Here's how the part is built. I have some questions about the finished solid (model axes, mm). A direction names the side the tool comes from. Coordinates: 2 decimals unless noted, no trailing zeros. Loops run counter-clockwise (first coordinate to the right, second up) from the corner with the lowest first, then second, coordinate; pieces in that order, holes last. Notation, with made-up numbers: (-14, 76) -> (33, 76) arc R8 cw to (33, 86) -> close; hole circle Ø11 at (-8, 27.5). An arc over 180 degrees is marked (long way). Use CSV: the item, a comma, the result in double quotes. Start each with the question number.
from build123d import *

# Parameters (mm, degrees)
SKETCH1_W           = 25.4
SKETCH1_H           = 299.72
BOSS_EXTRUDE1_DEPTH = 417.83
SKETCH2_W           = 223.52
SKETCH2_H           = 810.26
CUT_EXTRUDE1_DEPTH  = 19.05
SKETCH3_W           = 25.4
SKETCH3_H           = 118.11
CUT_EXTRUDE2_DEPTH  = 12.7


with BuildPart() as part:
    # Sketch1 → Boss-Extrude1 (new, symmetric)
    with BuildSketch(Plane(origin=(0, 0, 0), x_dir=(1, 0, 0), z_dir=(0, 1, 0))):
        Rectangle(SKETCH1_W, SKETCH1_H)
    extrude(amount=BOSS_EXTRUDE1_DEPTH, both=True)

    # Sketch2 → Cut-Extrude1 (cut)
    with BuildSketch(Plane(origin=(12.7, 0, 0), x_dir=(0, 0, -1), z_dir=(1, 0, 0))):
        Rectangle(SKETCH2_W, SKETCH2_H)
    extrude(amount=-CUT_EXTRUDE1_DEPTH, mode=Mode.SUBTRACT)

    # Sketch3 → Cut-Extrude2 (cut)
    with BuildSketch(Plane.ZY.offset(12.7)):
        with Locations((130.81, 231.775)):
            Rectangle(SKETCH3_W, SKETCH3_H)
    extrude(amount=-CUT_EXTRUDE2_DEPTH, mode=Mode.SUBTRACT)


solid = part.part
1) Which directions (+Z, -Z, +X, -X, +Y, -Y) give clear straight access to the entire face, cutting with the end or side of a thin tool? Please do faces 5 (the face through (3, -405.13, 2)), 6 (the face through (0, 6, -149.86)), 7 (the face through (0, 233, 131)).
2) Thinking about a two-plate mould opening in Y: for faces 1 (the face through (0, 417.83, -2)), 2 (the face through (3, -6, 111.76)), 3 (the face through (3, 405.13, 2)), 4 (the face through (-12.7, 6, 2)), which applies, pulls with the +Y half, pulls with the -Y half, needs draft (parallel to the pull), parting line crosses it, or undercut?
3) Please list where these lines run through material, in increasing order: L1, parallel to Z at x = -1.25, y = 341.5; L2, parallel to Y at x = 11.5, z = 6; L3, parallel to Z at x = -1, y = 262. Write a range as [from, to].
4) I want a section at B-B, the plane y = 279. Please give me the cut outline in (x, z).
5) I want a section at A-A, the plane z = -3.5. Please give me the cut outline in (x, y), plus the area to 3 significant figures.
6) For P1, Ø2, axis at y = -91, z = -99.5, coming from the +X side, with a flat end and sliding along its axis, tell me the tip position at first contact or that it passes through.
7) I want a section at C-C, the plane y = -154. Please give me the cut outline in (x, z).
Return value:
1,face 5,"+X"
1,face 6,"-Z, +X, -X, +Y, -Y"
1,face 7,"-X"
2,face 1,"pulls with the +Y half"
2,face 2,"undercut"
2,face 3,"undercut"
2,face 4,"needs draft"
3,L1,"z = [-149.86, -111.76], [111.76, 149.86]"
3,L2,"y = [-417.83, -405.13], [405.13, 417.83]"
3,L3,"z = [-149.86, -111.76], [111.76, 118.11], [143.51, 149.86]"
4,outline,"(-12.7, -149.86) -> (12.7, -149.86) -> (12.7, -111.76) -> (-6.35, -111.76) -> (-6.35, 111.76) -> (12.7, 111.76) -> (12.7, 149.86) -> (-12.7, 149.86) -> (-12.7, 143.51) -> (0, 143.51) -> (0, 118.11) -> (-12.7, 118.11) -> close"
5,outline,"(-12.7, -417.83) -> (12.7, -417.83) -> (12.7, -405.13) -> (-6.35, -405.13) -> (-6.35, 405.13) -> (12.7, 405.13) -> (12.7, 417.83) -> (-12.7, 417.83) -> close"
5,area,"5,790 mm²"
6,P1,"stops at x = -6.35"
7,outline,"(-12.7, -149.86) -> (12.7, -149.86) -> (12.7, -111.76) -> (-6.35, -111.76) -> (-6.35, 111.76) -> (12.7, 111.76) -> (12.7, 149.86) -> (-12.7, 149.86) -> close"
